For this review, take the finished solid that the model builds, in its own axes (mm). Face numbers are marked on the shaded views. A direction names the side the tool comes from. Give positions to 0.01 mm unless a question says otherwise; leave off trailing zeros. Order: outer loops, then holes, each group sorted by start corner. A loop starts at its lowest first (then second) coordinate and runs counter-clockwise, first axis right, second up.
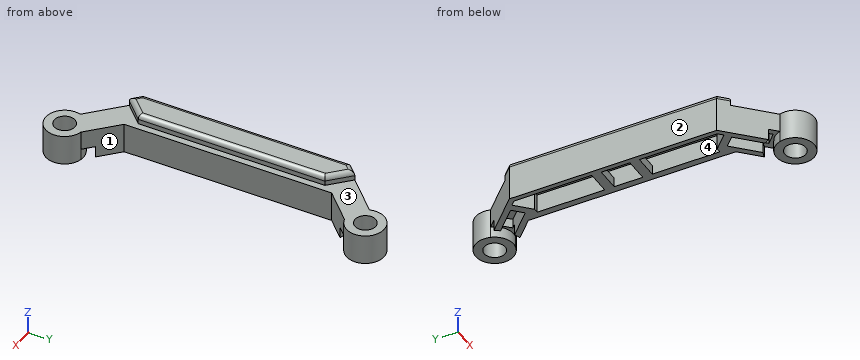
from build123d import *
from build123d.topology import SkipClean

# Parameters (mm, degrees)
EXTRUDE_1_DEPTH      = 3.2
SKETCH_2_R           = 1.1
CUT_EXTRUDE_1_DEPTH  = 3.2
EXTRUDE_2_DEPTH      = 1
FILLET_2_R           = 0.5
CUT_EXTRUDE_10_DEPTH = 3.7
SKETCH_9_W           = 0.5
SKETCH_9_H           = 19.185786438
CUT_EXTRUDE_11_DEPTH = 2
CUT_EXTRUDE_12_DEPTH = 3.2
CUT_EXTRUDE_13_DEPTH = 2.2
CUT_EXTRUDE_14_DEPTH = 1.2
SKETCH_15_W          = 2.5
SKETCH_15_H          = 1
EXTRUDE_3_DEPTH      = 1


with BuildPart() as part:
    # 草图1 → 凸台-拉伸1 (new body)
    with BuildSketch(Plane.XY):
        with BuildLine():
            Line((-6.2, 0), (-6.2, 10.9))
            Line((-6.2, 10.9), (-1.905985669, 15.194014331))
            ThreePointArc((-1.905985669, 15.194014331), (0.989561851, 17.538035484), (0.451668523, 13.851668523))
            Line((0.451668523, 13.851668523), (-2, 11.4))
            Line((-2, 11.4), (-2, 0))
            Line((-2, 0), (-2, -11.4))
            Line((-2, -11.4), (0.451668523, -13.851668523))
            ThreePointArc((0.451668523, -13.851668523), (0.989561851, -17.538035484), (-1.905985669, -15.194014331))
            Line((-1.905985669, -15.194014331), (-6.2, -10.9))
            Line((-6.2, -10.9), (-6.2, 0))
        make_face()
    extrude(amount=EXTRUDE_1_DEPTH)

    # 草图2 → 切除-拉伸1 (cut)
    with BuildSketch(Plane.XY.offset(3.2)):
        with Locations((0, 15.8)):
            Circle(SKETCH_2_R)
        with Locations((0, -15.8)):
            Circle(SKETCH_2_R)
    extrude(amount=-CUT_EXTRUDE_1_DEPTH, mode=Mode.SUBTRACT)

    # 草图3 → 凸台-拉伸2 (add)
    with BuildSketch(Plane.XY.offset(3.2)):
        Polygon((-3.2, 0), (-3.2, 9.8), (-5.25, 11.85), (-6.2, 10.9), (-6.2, -10.9), (-5.25, -11.85), (-3.2, -9.8), align=None)
    extrude(amount=EXTRUDE_2_DEPTH)

    # 圆角2
    fillet_2_edges = [part.edges().sort_by_distance(p)[0] for p in [
        (-4.225, -10.825, 4.2),
        (-5.725, -11.375, 4.2),
        (-3.2, 0, 4.2),
        (-4.225, 10.825, 4.2),
        (-5.725, 11.375, 4.2),
        (-6.2, 0, 4.2),
    ]]
    fillet(fillet_2_edges, radius=FILLET_2_R)

    # 草图7 → 切除-拉伸10 (cut)
    with BuildSketch(Plane.XY):
        Polygon((-5.25, 11.142893219), (-3.7, 9.592893219), (-3.7, -9.592893219), (-5.25, -11.142893219), (-5.7, -10.692893219), (-5.7, 10.692893219), align=None)
    extrude(amount=CUT_EXTRUDE_10_DEPTH, mode=Mode.SUBTRACT)

    # 草图9 → 切除-拉伸11 (cut)
    with BuildSketch(Plane(origin=(0, 0, 0), x_dir=(-1, 0, 0), z_dir=(0, 0, -1))):
        with Locations((3.45, 0)):
            Rectangle(SKETCH_9_W, SKETCH_9_H)
    extrude(amount=-CUT_EXTRUDE_11_DEPTH, mode=Mode.SUBTRACT)

    # 草图10 → 切除-拉伸12 (cut)
    with BuildSketch(Plane.XY.offset(3.2)):
        Polygon((-2.5, 10.9), (-2.5, -10.9), (-2, -11.4), (-2, 11.4), align=None)
    extrude(amount=-CUT_EXTRUDE_12_DEPTH, mode=Mode.SUBTRACT)

    # 草图12 → 切除-拉伸13 (cut)
    with BuildSketch(Plane(origin=(0, 0, 0), x_dir=(-1, 0, 0), z_dir=(0, 0, -1))):
        Polygon((3.63137085, 10.617157288), (4.632842712, 11.61862915), (1.804415588, 14.447056275), (0.802943725, 13.445584413), align=None)
        Polygon((1.804415588, -14.447056275), (0.802943725, -13.445584413), (3.63137085, -10.617157288), (4.632842712, -11.61862915), align=None)
    extrude(amount=-CUT_EXTRUDE_13_DEPTH, mode=Mode.SUBTRACT)

    # 草图14 → 切除-拉伸14 (cut)
    with SkipClean():  # the faces are left unmerged after this step: merging them gives an invalid solid
        with BuildSketch(Plane(origin=(0, 0, 0), x_dir=(-1, 0, 0), z_dir=(0, 0, -1))):
            with BuildLine():
                Line((1.905985669, -15.194014331), (2.669282051, -14.430717949))
                ThreePointArc((2.669282051, -14.430717949), (1.792734548, -13.394568055), (0.549285568, -12.850714432))
                Line((0.549285568, -12.850714432), (-0.451668523, -13.851668523))
                ThreePointArc((-0.451668523, -13.851668523), (0.989561851, -14.061964516), (1.905985669, -15.194014331))
            make_face()
            with BuildLine():
                Line((-0.451668523, 13.851668523), (0.549285568, 12.850714432))
                ThreePointArc((0.549285568, 12.850714432), (1.792734548, 13.394568055), (2.669282051, 14.430717949))
                Line((2.669282051, 14.430717949), (1.905985669, 15.194014331))
                ThreePointArc((1.905985669, 15.194014331), (0.989561851, 14.061964516), (-0.451668523, 13.851668523))
            make_face()
        extrude(amount=-CUT_EXTRUDE_14_DEPTH, mode=Mode.SUBTRACT)

    # 草图15 → 凸台-拉伸3 (add)
    with SkipClean():  # the faces are left unmerged after this step: merging them gives an invalid solid
        with BuildSketch(Plane(origin=(0, 0, 0), x_dir=(-1, 0, 0), z_dir=(0, 0, -1))):
            with Locations((4.45, 2)):
                Rectangle(SKETCH_15_W, SKETCH_15_H)
            with Locations((4.45, -2)):
                Rectangle(SKETCH_15_W, SKETCH_15_H)
        extrude(amount=-EXTRUDE_3_DEPTH)


solid = part.part
1) We need section A-A on y = 15.8. Give the boundary of the cut face in (x, z), then the cut area to 3 significant figures.
Answer sheet:
outline: (-2, 0) - (-1.1, 0) - (-1.1, 3.2) - (-2, 3.2) - close; (1.1, 0) - (2, 0) - (2, 3.2) - (1.1, 3.2) - close
area: 5.76 mm2
2) Clearance check with flat-ended pins moving along their axes: pin 1 (0.6 mm diameter, centred on x = -4.5, y = -4, fed in from -Z); pin 2 (0.5 mm diameter, centred on x = -4, z = 0.5, fed in from -Y); pin 3 (1.1 mm diameter, centred on x = -4, z = 0.5, fed in from +Y). State where each tip first meets the part, or that it passes through.
Answer sheet:
pin 1: stops at z = 3.7
pin 2: stops at y = -13.35
pin 3: stops at y = 13.65
3) We need section B-B on x = 0. Give the boundary of the cut face in (y, z), then the cut area to 3 significant figures.
Answer sheet:
outline: (-17.8, 0) - (-16.9, 0) - (-16.9, 3.2) - (-17.8, 3.2) - close; (-14.7, 0) - (-13.8, 0) - (-13.8, 1.2) - (-13.4, 1.2) - (-13.4, 3.2) - (-14.7, 3.2) - close; (13.4, 1.2) - (13.8, 1.2) - (13.8, 0) - (14.7, 0) - (14.7, 3.2) - (13.4, 3.2) - close; (16.9, 0) - (17.8, 0) - (17.8, 3.2) - (16.9, 3.2) - close
area: 13.1 mm2
4) We need section D-D on y = 4. Give the boundary of the cut face in (x, z).
Answer sheet:
outline: (-6.2, 0) - (-5.7, 0) - (-5.7, 3.7) - (-3.7, 3.7) - (-3.7, 2) - (-3.2, 2) - (-3.2, 0) - (-2.5, 0) - (-2.5, 3.2) - (-3.2, 3.2) - (-3.2, 3.7) arc R0.5 ccw to (-3.7, 4.2) - (-5.7, 4.2) arc R0.5 ccw to (-6.2, 3.7) - close
5) We need section C-C on z = 1.5. Give the boundary of the cut face in (x, y), then the cut area to 3 significant figures.
Answer sheet:
outline: (-6.2, -10.9) - (-1.91, -15.19) arc R2 ccw (long way) to (0.45, -13.85) - (-2.5, -10.9) - (-2.5, 10.9) - (0.45, 13.85) arc R2 ccw (long way) to (-1.91, 15.19) - (-6.2, 10.9) - close; hole (-5.7, -10.69) - (-5.25, -11.14) - (-3.7, -9.59) - (-3.2, -9.59) - (-3.2, 9.59) - (-3.7, 9.59) - (-5.25, 11.14) - (-5.7, 10.69) - close; hole (-4.63, -11.62) - (-1.8, -14.45) - (-0.8, -13.45) - (-3.63, -10.62) - close; hole (-4.63, 11.62) - (-3.63, 10.62) - (-0.8, 13.45) - (-1.8, 14.45) - close; hole circle Ø2.2 at (0, -15.8); hole circle Ø2.2 at (0, 15.8)
area: 60.1 mm2
6) Tool access review of the marked faces 1 and 2: name each direction out of +Z, -Z, +X, -X, +Y, -Y from which nothing blocks a thin tool from reaching the whole face with its end or side.
Answer sheet:
face 1: +Z, -Z, +X
face 2: +Z, -Z, -X, +Y, -Y
7) Draft analysis for pull direction Y (two halves, no side actions). For the marked faces 3 and 4, state which applies: +Y half, -Y half, draft (parallel to the pull), parting line (faces both ways), or undercut.
Answer sheet:
face 3: draft
face 4: undercut
8) To check wall thickness, follow line 1 (Y direction, x = 0, z = 0.75); line 2 (X direction, y = -4, z = 2.35); line 3 (Y direction, x = -0.75, z = 0.7). State the ranges of each line that lie inside material, in increasing order.
Answer sheet:
line 1: y = -17.8 to -16.9, -14.7 to -13.8, 13.8 to 14.7, 16.9 to 17.8
line 2: x = -6.2 to -5.7, -3.7 to -2.5
line 3: y = -17.65 to -16.6, -15 to -13.95, -12.9 to -12.65, 12.65 to 12.9, 13.95 to 15, 16.6 to 17.65
